```python
from build123d import *

# Parameters (mm, degrees)
SKETCH1_W           = 76.2
SKETCH1_H           = 76.2
BOSS_EXTRUDE1_DEPTH = 15.875
SKETCH2_R           = 3.175
CUT_EXTRUDE1_DEPTH  = 109.92610167
SKETCH2_3_R         = 3.175
CUT_EXTRUDE2_DEPTH  = 109.92610167


with BuildPart() as part:
    # Sketch1 → Boss-Extrude1 (new body)
    with BuildSketch(Plane(origin=(0, 0, 0), x_dir=(1, 0, 0), z_dir=(0, 1, 0))):
        with Locations((38.1, 38.1)):
            Rectangle(SKETCH1_W, SKETCH1_H)
    extrude(amount=BOSS_EXTRUDE1_DEPTH)

    # Sketch2 → Cut-Extrude1 (cut, through all)
    with BuildSketch(Plane(origin=(0, 15.875, 0), x_dir=(1, 0, 0), z_dir=(0, 1, 0))):
        with Locations(Location((38.1, 70.00228824, 0), (0, 0, 270))):
            Circle(SKETCH2_R)
        with Locations(Location((38.1, 6.19771176, 0), (0, 0, 270))):
            Circle(SKETCH2_R)
    extrude(amount=-CUT_EXTRUDE1_DEPTH, mode=Mode.SUBTRACT)

    # Sketch2_3 → Cut-Extrude2 (cut, through all)
    with BuildSketch(Plane(origin=(0, 15.875, 0), x_dir=(1, 0, 0), z_dir=(0, 1, 0))):
        with Locations(Location((9.4996, 38.1, 0), (0, 0, 270))):
            Circle(SKETCH2_3_R)
        with Locations(Location((66.7004, 38.1, 0), (0, 0, 270))):
            Circle(SKETCH2_3_R)
    extrude(amount=-CUT_EXTRUDE2_DEPTH, mode=Mode.SUBTRACT)


solid = part.part
```
The model under review builds one solid part; all positions refer to its coordinate system, in mm. Round coordinates to 2 decimals unless told otherwise and drop trailing zeros. Write each loop counter-clockwise with the first axis right and the second up, starting at its lowest first coordinate (ties: lowest second). Pieces come first, ordered by that corner, then holes. Notation, with made-up numbers: M 13.25,4.5 L 21.25,4.5 A27 cw 21.25,20.5 Z; hole C -30,78 d2. An arc over 180 degrees is marked long. Use CSV: the item, a comma, the result in double quotes. Start each with the question number.
(1) The part is to be moulded in two halves that separate along X. For faces 1 (the face through (0, 8, -38)), 2 (the face through (76.2, 8, -38)), 3 (the face through (11.645, 8.049, -40.44)), say which applies: +X half, -X half, draft (parallel to the pull), parting line (faces both ways), or undercut.
(2) For line 1 along X through (y, z) = (10, -38.1); line 2 along X through (y, z) = (8.5, -37); line 3 along Z through (x, y) = (10, 1.5), list the stretches that pass through material, from the lowest coordinate up.
(3) Clearance check with a flat-ended pin moving along its axis: P1, Ø4, axis at x = 15, z = -53.5, coming from the -Y side. State where the tip first meets the part, or that it passes through.
(4) We need section A-A, the plane z = -38.1. State the section outline as (x, y) points (3 decimals), then the cut area to 3 significant figures.
(5) We need section B-B, the plane x = 38.1. State the section outline as (y, z) points (3 decimals).
Findings:
1,face 1,"-X half"
1,face 2,"+X half"
1,face 3,"undercut"
2,line 1,"0 to 6.32, 12.67 to 63.53, 69.88 to 76.2"
2,line 2,"0 to 6.52, 12.48 to 63.72, 69.68 to 76.2"
2,line 3,"-76.2 to -41.24, -34.96 to 0"
3,P1,"y = 0"
4,outline,"M 0,0 L 6.325,0 L 6.325,15.875 L 0,15.875 Z; M 12.675,0 L 63.525,0 L 63.525,15.875 L 12.675,15.875 Z; M 69.875,0 L 76.2,0 L 76.2,15.875 L 69.875,15.875 Z"
4,area,"1,010 mm^2"
5,outline,"M 0,-76.2 L 15.875,-76.2 L 15.875,-73.177 L 0,-73.177 Z; M 0,-66.827 L 15.875,-66.827 L 15.875,-9.373 L 0,-9.373 Z; M 0,-3.023 L 15.875,-3.023 L 15.875,0 L 0,0 Z"
